```python
from build123d import *

# Parameters (mm, degrees)
F0_R     = 58.18106
F1_DEPTH = 103.465883
F2_R     = 13.503073
F3_DEPTH = 177.737946
F4_DEPTH = 213.257074


with BuildPart() as f1:
    # F0 (on Front) → F1 (new body)
    with BuildSketch(Plane.XZ):
        Circle(F0_R)
    extrude(amount=F1_DEPTH)

    # F2 (on face) → F3 (cut)
    with BuildSketch(Plane.XZ.offset(103.465883)):
        with Locations((8.346159, 33.583872)):
            Circle(F2_R)
    extrude(amount=-F3_DEPTH, mode=Mode.SUBTRACT)

    # F2 (on face) → F4 (cut)
    with BuildSketch(Plane.XZ.offset(103.465883)):
        with Locations((-29.361053, 18.31566)):
            Circle(F2_R)
        with Locations((-26.492292, -22.264171)):
            Circle(F2_R)
        with Locations((12.987918, -32.075673)):
            Circle(F2_R)
        with Locations((34.519265, 2.440317)):
            Circle(F2_R)
    extrude(amount=-F4_DEPTH, mode=Mode.SUBTRACT)


solid = f1.part
```
Check sheet for the modelled part. Datum: model origin and axes. Units: mm. Round coordinates to 2 decimals unless told otherwise and drop trailing zeros. Loops run counter-clockwise (first coordinate to the right, second up) from the corner with the lowest first, then second, coordinate; pieces in that order, holes last. Notation, with made-up numbers: (81, 55) -> (86, 55) arc R16 ccw to (86, 68) -> close; hole circle Ø8 at (-11.5, 83). An arc over 180 degrees is marked (long way). Write item = value, one per line. Start each with the question number.
1) Release check for a two-part mould opening along X. For faces 1 (the cylindrical face through (23.804, -52.457, -5.776)), 2 (the cylindrical face through (-12.6, -51, -56.8)), 3 (the cylindrical face through (11.23, -52.457, -18.688)), 4 (the flat face through (-1, -103.466, 1)) record: released by +X, released by -X, zero draft, split by the parting line, or undercut.
2) Sectioned sample at C-C, the plane z = 41.5. Record the cut outline in (x, y), plus the area to 3 significant figures.
3) Gauge pin test, flat ends, axial feed: pin 1 Ø3 at (x, y) = (-1, -51.5) entering from +Z; pin 2 Ø8 at (y, z) = (-81, -27) entering from +X; pin 3 Ø3 at (x, y) = (3, -60) entering from -Z; pin 4 Ø24.5 at (x, z) = (12.99, -32.08) entering from +Y. Record the tip position at first contact, or that the pin passes through.
4) Thickness scan on probe 1 along X at (y, z) = (-27, -27); probe 2 along Z at (x, y) = (13, -91); probe 3 along Z at (x, y) = (-37, -43). Record the ranges inside material, lowest first.
5) Sectioned sample at D-D, the plane y = -14. Record the cut outline in (x, z).
6) Sectioned sample at B-B, the plane x = -28.5. Record the cut outline in (y, z).
7) Sectioned sample at A-A, the plane z = -26.5. Record the cut outline in (x, y), plus the area to 3 significant figures.
Results are:
q1.face_1 = undercut
q1.face_2 = split by the parting line
q1.face_3 = undercut
q1.face_4 = zero draft
q2.outline = (-40.78, -103.47) -> (-2.59, -103.47) -> (-2.59, 0) -> (-40.78, 0) -> close; (19.29, -103.47) -> (40.78, -103.47) -> (40.78, 0) -> (19.29, 0) -> close
q2.area = 6,170 mm^2
q3.pin_1 = 58.18
q3.pin_2 = 53.44
q3.pin_3 = -58.16
q3.pin_4 = through
q4.probe_1 = -51.54 to -39.14, -13.85 to 0.48, 25.5 to 51.54
q4.probe_2 = -56.71 to -45.58, -18.57 to 20.91, 46.26 to 56.71
q4.probe_3 = -44.9 to -30.74, -13.78 to 7.18, 29.45 to 44.9
q5.outline = circle Ø116.36 at (0, 0); hole circle Ø27.01 at (-29.36, 18.32); hole circle Ø27.01 at (-26.49, -22.26); hole circle Ø27.01 at (8.35, 33.58); hole circle Ø27.01 at (12.99, -32.08); hole circle Ø27.01 at (34.52, 2.44)
q6.outline = (-103.47, -50.72) -> (0, -50.72) -> (0, -35.62) -> (-103.47, -35.62) -> close; (-103.47, -8.91) -> (0, -8.91) -> (0, 4.84) -> (-103.47, 4.84) -> close; (-103.47, 31.79) -> (0, 31.79) -> (0, 50.72) -> (-103.47, 50.72) -> close
q7.outline = (-51.8, -103.47) -> (-39.31, -103.47) -> (-39.31, 0) -> (-51.8, 0) -> close; (-13.67, -103.47) -> (0.69, -103.47) -> (0.69, 0) -> (-13.67, 0) -> close; (25.29, -103.47) -> (51.8, -103.47) -> (51.8, 0) -> (25.29, 0) -> close
q7.area = 5,520 mm^2
